from build123d import *

# Parameters (mm, degrees)
SKETCH1_R                = 76.2
SKETCH1_R_2              = 73.7
BOSS_EXTRUDE1_DEPTH      = 260
BOSS_EXTRUDE2_DEPTH      = 1.5
BOSS_EXTRUDE2_DEPTH_BACK = 1.5
BOSS_EXTRUDE3_DEPTH      = 1.5
BOSS_EXTRUDE3_DEPTH_BACK = 1.5
SKETCH4_W                = 2
SKETCH4_H                = 260
CIRPATTERN1_COUNT        = 4
SKETCH6_R                = 73.7
BOSS_EXTRUDE4_DEPTH      = 10
CHAMFER1_START           = 264.638732699
CHAMFER1_2_OUTLINE_R     = 76.2
CHAMFER1_2_OUTLINE_R_2   = 73.7
CHAMFER1_2_DEPTH         = 5.361267301
CHAMFER1_START_2         = 258
CHAMFER1_3_DEPTH         = 2


with BuildPart() as part:
    # Sketch1 → Boss-Extrude1 (new body)
    with BuildSketch(Plane(origin=(0, 0, 0), x_dir=(1, 0, 0), z_dir=(0, 1, 0))):
        with Locations(Location((0, 0, 0), (0, 0, 270))):
            Circle(SKETCH1_R)
        with Locations(Location((0, 0, 0), (0, 0, 270))):
            Circle(SKETCH1_R_2, mode=Mode.SUBTRACT)
    extrude(amount=BOSS_EXTRUDE1_DEPTH)



with BuildPart() as body_2:
    # Sketch2 → Boss-Extrude2 (new, two sides: drawn at the far end of the back side and taken through both)
    with BuildSketch(Plane.XY.offset(-BOSS_EXTRUDE2_DEPTH_BACK)):
        Polygon((76.2, 0), (76.2, 260), (246.2, 120), (246.2, 0), align=None)
    extrude(amount=BOSS_EXTRUDE2_DEPTH + BOSS_EXTRUDE2_DEPTH_BACK)


with BuildPart() as part_1:
    add(part.part)

    add(body_2.part)  # Boss-Extrude3 merges body 2
    # Sketch4 → Boss-Extrude3 (add, two sides: drawn at the far end of the back side and taken through both)
    with BuildSketch(Plane.XY.offset(-BOSS_EXTRUDE3_DEPTH_BACK)):
        with Locations((75.2, 130)):
            Rectangle(SKETCH4_W, SKETCH4_H)
    extrude(amount=BOSS_EXTRUDE3_DEPTH + BOSS_EXTRUDE3_DEPTH_BACK)


with BuildPart() as cirpattern1_1:
    # CirPattern1: pattern copy
    add(part_1.part.rotate(Axis((0, 0, 0), (0, 1, 0)), 1 * 360 / CIRPATTERN1_COUNT))


with BuildPart() as cirpattern1_2:
    # CirPattern1: pattern copy
    add(part_1.part.rotate(Axis((0, 0, 0), (0, 1, 0)), 2 * 360 / CIRPATTERN1_COUNT))


with BuildPart() as cirpattern1_3:
    # CirPattern1: pattern copy
    add(part_1.part.rotate(Axis((0, 0, 0), (0, 1, 0)), 3 * 360 / CIRPATTERN1_COUNT))


with BuildPart() as part_2:
    add(part_1.part)

    add(cirpattern1_1.part)  # Boss-Extrude4 merges CirPattern1_1

    add(cirpattern1_2.part)  # Boss-Extrude4 merges CirPattern1_2

    add(cirpattern1_3.part)  # Boss-Extrude4 merges CirPattern1_3
    # Sketch6 → Boss-Extrude4 (add)
    with BuildSketch(Plane(origin=(0, 260, 0), x_dir=(1, 0, 0), z_dir=(0, 1, 0))):
        with BuildLine():
            ThreePointArc((76.18523479, -1.5), (76.2, 0), (76.18523479, 1.5))
            ThreePointArc((76.18523479, 1.5), (53.881536726, 53.881536726), (1.5, 76.18523479))
            ThreePointArc((1.5, 76.18523479), (0, 76.2), (-1.5, 76.18523479))
            ThreePointArc((-1.5, 76.18523479), (-53.881536726, -53.881536726), (76.18523479, -1.5))
        make_face()
        with Locations(Location((0, 0, 0), (0, 0, 270))):
            Circle(SKETCH6_R, mode=Mode.SUBTRACT)
    extrude(amount=BOSS_EXTRUDE4_DEPTH)

    # Chamfer1: read off the stored shape, not the designer's step
    # Chamfer1 outline → Chamfer1 (revolve, cut)
    with BuildSketch(Plane.XY):
        Polygon((73.7, 264.638732699), (76.2, 259.277465397), (76.2, 264.638732699), align=None)
    revolve(axis=Axis((0, 0, 0), (0, 1, 0)), mode=Mode.SUBTRACT)

    # Chamfer1 2 outline → Chamfer1 2 (cut)
    with BuildSketch(Plane(origin=(0, 0, 0), x_dir=(1, 0, 0), z_dir=(0, 1, 0)).offset(CHAMFER1_START)):
        Circle(CHAMFER1_2_OUTLINE_R)
        Circle(CHAMFER1_2_OUTLINE_R_2, mode=Mode.SUBTRACT)
    extrude(amount=CHAMFER1_2_DEPTH, mode=Mode.SUBTRACT)

    # Chamfer1 3 outline → Chamfer1 3 (add)
    with BuildSketch(Plane(origin=(0, 0, 0), x_dir=(1, 0, 0), z_dir=(0, 1, 0)).offset(CHAMFER1_START_2)):
        with BuildLine():
            ThreePointArc((76.18523479, -1.5), (76.2, 0), (76.18523479, 1.5))
            Line((76.18523479, 1.5), (75.848245783, 1.5))
            ThreePointArc((75.848245783, 1.5), (75.863076582, 0), (75.848245783, -1.5))
            Line((75.848245783, -1.5), (76.18523479, -1.5))
        make_face()
        with BuildLine():
            Line((1.5, 75.848245783), (1.5, 76.18523479))
            ThreePointArc((1.5, 76.18523479), (0, 76.2), (-1.5, 76.18523479))
            Line((-1.5, 76.18523479), (-1.5, 75.848245783))
            ThreePointArc((-1.5, 75.848245783), (0, 75.863076582), (1.5, 75.848245783))
        make_face()
        with BuildLine():
            ThreePointArc((-1.5, -76.18523479), (0, -76.2), (1.5, -76.18523479))
            Line((1.5, -76.18523479), (1.5, -75.848245783))
            ThreePointArc((1.5, -75.848245783), (0, -75.863076582), (-1.5, -75.848245783))
            Line((-1.5, -75.848245783), (-1.5, -76.18523479))
        make_face()
        with BuildLine():
            Line((-75.848245783, 1.5), (-76.18523479, 1.5))
            ThreePointArc((-76.18523479, 1.5), (-76.2, 0), (-76.18523479, -1.5))
            Line((-76.18523479, -1.5), (-75.848245783, -1.5))
            ThreePointArc((-75.848245783, -1.5), (-75.863076582, 0), (-75.848245783, 1.5))
        make_face()
    extrude(amount=CHAMFER1_3_DEPTH)


solid = part_2.part
Input: part model. Units: mm. Frame: model coordinates. A direction names the side the tool comes from. Give positions to 0.01 mm unless a question says otherwise; leave off trailing zeros. Write each loop counter-clockwise with the first axis right and the second up, starting at its lowest first coordinate (ties: lowest second). Pieces come first, ordered by that corner, then holes. Notation, with made-up numbers: M -23.75,-22.5 L 18.25,-22.5 A17 ccw 18.25,-2.5 Z; hole C 10,-9 d11. An arc over 180 degrees is marked long. Use one line per item in the form item = value.
1. Cut plane A-A on y = 95.5. Return loops of the section in (x, z).
Outcome:
outline = M -246.2,-1.5 L -76.19,-1.5 A76.2 ccw -1.5,-76.19 L -1.5,-246.2 L 1.5,-246.2 L 1.5,-76.19 A76.2 ccw 76.19,-1.5 L 246.2,-1.5 L 246.2,1.5 L 76.19,1.5 A76.2 ccw 1.5,76.19 L 1.5,246.2 L -1.5,246.2 L -1.5,76.19 A76.2 ccw -76.19,1.5 L -246.2,1.5 Z; hole C 0,0 d147.4
2. Cut plane B-B on y = 207.5. Return loops of the section in (x, z), and give its area (3 significant figures).
Outcome:
outline = M -139.95,-1.5 L -76.19,-1.5 A76.2 ccw -1.5,-76.19 L -1.5,-139.95 L 1.5,-139.95 L 1.5,-76.19 A76.2 ccw 76.19,-1.5 L 139.95,-1.5 L 139.95,1.5 L 76.19,1.5 A76.2 ccw 1.5,76.19 L 1.5,139.95 L -1.5,139.95 L -1.5,76.19 A76.2 ccw -76.19,1.5 L -139.95,1.5 Z; hole C 0,0 d147.4
area = 1,940 mm²
3. Reachability of faces 4 (the face through (-143, 99, 1.5)), 5 (the face through (143, 99, -1.5)), 6 (the face through (-72, 0, 17)), 7 (the face through (-160, 99, -1.5)), 8 (the face through (1.5, 99, 143)) from +Z, -Z, +X, -X, +Y, -Y: full face, straight path, thin tool, end or side. Return the list, or none.
Outcome:
face_4 = +Z, -X, +Y, -Y
face_5 = -Z, +X, +Y, -Y
face_6 = +Z, -Z, +X, -X, -Y
face_7 = -Z, -X, +Y, -Y
face_8 = +Z, +X, +Y, -Y
4. Cut plane D-D on x = -152. Return loops of the section in (y, z), and give its area (3 significant figures).
Outcome:
outline = M 0,-1.5 L 197.58,-1.5 L 197.58,1.5 L 0,1.5 Z
area = 593 mm²
5. Mould query, pull axis X, two halves, no side actions, for faces 1 (the face through (22.137, 130.467, 70.297)), 2 (the face through (-1.5, 99, -143)), 3 (the face through (1.5, 99, -160)). Classes: released by +X, released by -X, zero draft, split by the parting line, or undercut.
Outcome:
face_1 = undercut
face_2 = released by -X
face_3 = released by +X
6. First-contact query: P1, Ø5, axis at y = 131, z = -91.5, coming from the +X side; P2, Ø6, axis at x = -8.5, y = 137, coming from the +Z side; P3, Ø10, axis at y = 59.5, z = -156.5, coming from the -X side. Flat tips, straight axial feed; report the tip coordinate or a pass-through.
Outcome:
P1 = 1.5
P2 = 76
P3 = -1.5
7. Ray query, L1, parallel to X at y = 106, z = 0; L2, parallel to X at y = 119, z = -148.5. Return the intervals inside material, ascending.
Outcome:
L1 = -246.2 to -73.7, 73.7 to 246.2
L2 = -1.5 to 1.5
8. Cut plane C-C on z = 102.5. Return loops of the section in (x, y).
Outcome:
outline = M -1.5,0 L 1.5,0 L 1.5,238.34 L -1.5,238.34 Z
